Check sheet for the modelled part. Datum: model origin and axes. Units: mm. Face numbers are marked on the shaded views. Give positions to 0.01 mm unless a question says otherwise; leave off trailing zeros. Loops run counter-clockwise (first coordinate to the right, second up) from the corner with the lowest first, then second, coordinate; pieces in that order, holes last. Notation, with made-up numbers: M 64,81 L 70,81 A17 ccw 70,101 Z; hole C -14.75,73.25 d10. An arc over 180 degrees is marked long. Put each result on its own line as item: value. Start each with the question number.
```python
from build123d import *

# Parameters (mm, degrees)
F0_R     = 38.1
F1_DEPTH = 50.8
F2_R     = 31.75
F3_DEPTH = 45.212
F4_R     = 34.29
F5_DEPTH = 5.08
F6_W     = 73.66
F6_H     = 10.16
F7_DEPTH = 5.08
F8_R     = 36.83
F9_DEPTH = 2.286


with BuildPart() as f1:
    # F0 (on Right) → F1 (new body)
    with BuildSketch(Plane.YZ):
        Circle(F0_R)
    extrude(amount=F1_DEPTH)

    # F2 (on face) → F3 (cut)
    with BuildSketch(Plane.YZ.offset(50.8)):
        Circle(F2_R)
    extrude(amount=-F3_DEPTH, mode=Mode.SUBTRACT)

    # F4 (on face) → F5 (cut)
    with BuildSketch(Plane.YZ.offset(50.8)):
        Circle(F4_R)
    extrude(amount=-F5_DEPTH, mode=Mode.SUBTRACT)

    # F6 (on face) → F7 (cut)
    with BuildSketch(Plane.YZ.offset(50.8)):
        Rectangle(F6_W, F6_H)
    extrude(amount=-F7_DEPTH, mode=Mode.SUBTRACT)

    # F8 (on face) → F9 (cut)
    with BuildSketch(Plane.YZ.offset(45.72)):
        Circle(F8_R)
    extrude(amount=-F9_DEPTH, mode=Mode.SUBTRACT)


solid = f1.part
```
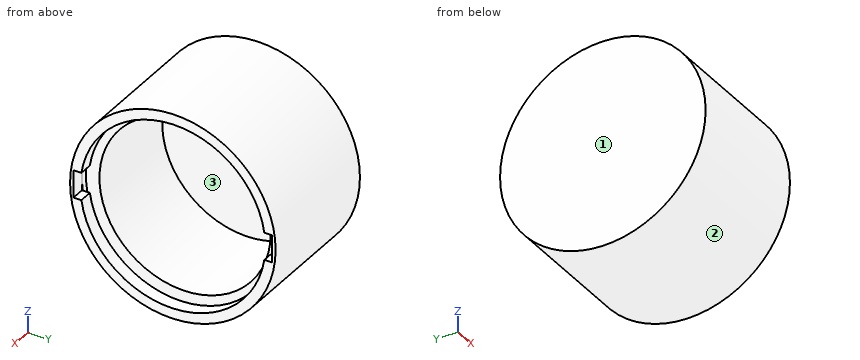
Q1. Section check B-B, the plane y = 0. Record the cut outline in (x, z).
Q2. Section check D-D, the plane y = 22. Record the cut outline in (x, z), then the cut area to 3 significant figures.
Q3. Section check A-A, the plane x = 48. Record the cut outline in (y, z).
Q4. Mould release check, pull along Z, two halves, no side actions. Record for the marked faces 1, 2 and 3: pulls with the +Z half, pulls with the -Z half, needs draft (parallel to the pull), parting line crosses it, or undercut.
Q5. Thickness scan on line 1 along Z through (x, y) = (44, 0); line 2 along Z through (x, y) = (17, 0); line 3 along X through (y, z) = (22.5, -28). Record the ranges inside material, lowest first. Write a range as [from, to].
Q6. Section check C-C, the plane x = 32. Record the cut outline in (y, z).
Q7. Depth check by flat-ended pin: P1, Ø4, axis at x = 17.5, z = 28, coming from the -Y side; P2, Ø10, axis at x = 5.5, y = -20, coming from the +Z side; P3, Ø1.5, axis at x = 47.5, z = 2, coming from the -Y side. Enter the tip coordinate at first touch or a pass-through.
Found:
1. outline: M 0,-38.1 L 50.8,-38.1 L 50.8,-34.29 L 45.72,-34.29 L 45.72,-36.83 L 43.43,-36.83 L 43.43,-31.75 L 5.59,-31.75 L 5.59,31.75 L 43.43,31.75 L 43.43,36.83 L 45.72,36.83 L 45.72,34.29 L 50.8,34.29 L 50.8,38.1 L 0,38.1 Z
2. outline: M 0,-31.11 L 50.8,-31.11 L 50.8,-26.3 L 45.72,-26.3 L 45.72,-29.54 L 43.43,-29.54 L 43.43,-22.89 L 5.59,-22.89 L 5.59,22.89 L 43.43,22.89 L 43.43,29.54 L 45.72,29.54 L 45.72,26.3 L 50.8,26.3 L 50.8,31.11 L 0,31.11 Z
2. area: 1,030 mm^2
3. outline: C 0,0 d76.2; hole M -36.83,-5.08 L -33.91,-5.08 A34.29 ccw 33.91,-5.08 L 36.83,-5.08 L 36.83,5.08 L 33.91,5.08 A34.29 ccw -33.91,5.08 L -36.83,5.08 Z
4. face 1: needs draft
4. face 2: parting line crosses it
4. face 3: undercut
5. line 1: z = [-38.1, -36.83], [36.83, 38.1]
5. line 2: z = [-38.1, -31.75], [31.75, 38.1]
5. line 3: x = [0, 43.43], [45.72, 50.8]
6. outline: C 0,0 d76.2; hole C 0,0 d63.5
7. P1: stops at y = -27.85
7. P2: stops at z = 35.02
7. P3: stops at y = -38.08
